Could you check a few things on this model? Use its own coordinates, in mm. A direction names the side the tool comes from. Give positions to 0.01 mm unless a question says otherwise; leave off trailing zeros. Loops run counter-clockwise (first coordinate to the right, second up) from the corner with the lowest first, then second, coordinate; pieces in that order, holes last. Notation, with made-up numbers: M 39,85 L 50,85 A11 cw 50,90 Z; hole C 10.5,6.25 d2. An arc over 180 degrees is marked long. Use CSV: the item, a comma, the result in double quotes.
Autodesk Inventor part; units mm, degrees
ref_plane "Work Plane1" through (0, -7, 0) normal (0, -1, 0) x (1, 0, 0)
ref_plane "YZ Plane" through (0, 0, 0) normal (1, 0, 0) x (0, 1, 0)
ref_plane "XZ Plane" through (0, 0, 0) normal (0, 1, 0) x (-1, 0, 0)
sketch "Sketch1" plane through (0, 0, 0) normal (0, 1, 0) x (-1, 0, 0)
  line L0 (0, 0) -> (3, 0)
  line L1 (3, 0) -> (3, -3)
  line L2 (0, 0) -> (-48.04, 0)
  line L3 (-48.04, 0) -> (-54, 0)
  line L4 (3, -3) -> (-54, -3)
  line L5 (-54, -3) -> (-54, 45)
  line L6 (-54, 45) -> (3, 45)
  line L7 (3, 45) -> (3, -3)
  line L8 (3, 21) -> (6.1215, 21)
  circle A0 centre (0, 0) radius 1.65
  circle A1 centre (-48.04, 0) radius 1.65
  line L9 (0, 42) -> (-48.04, 42)
  circle A2 centre (0, 42) radius 1.65
  circle A3 centre (-48.04, 42) radius 1.65
  line L10 (-54, -3) -> (-54, 8.785)
  line L11 (-54, 8.785) -> (-9.9, 8.785)
  line L12 (-9.9, 8.785) -> (-9.9, 23.785)
  line L13 (-9.9, 23.785) -> (-54, 23.785)
  dimension "d0" = 3
  dimension "d1" = 3
  dimension "d2" = 48.04
  dimension "d3" = 5.96
  dimension "d4" = 48
  dimension "d5" = 3.3
  dimension "d6" = 3.3
  dimension "d7" = 11.785
  dimension "d8" = 44.1
  dimension "d9" = 15
extrude "Extrusion1" add sketch "Sketch1" along normal blind 2 contours A0 L2 A1 L3 L5 L11 L12 L13 L6 L7 L0 | L0 L1 L4 L5 L3 A1 L2 A0
sketch "Sketch2" plane through (0, 0, 0) normal (0, -1, 0) x (1, 0, 0)
  line L0 (-3, -3) -> (-3, 45)
  line L1 (-3, -3) -> (-3, 5)
  line L2 (54, 8.785) -> (54, -3)
  line L3 (9.9, 8.785) -> (54, 8.785)
  line L4 (54, 8.785) -> (54, 4.785)
  line L5 (54, 8.785) -> (54, -3)
  line L6 (54, 23.785) -> (54, 27.785)
  line L7 (54, 45) -> (54, 23.785)
  line L8 (54, 27.785) -> (-3, 27.785)
  line L9 (-3, 5) -> (-3, 27.785)
  line L10 (9.9, 8.785) -> (54, 8.785)
  line L11 (54, 8.785) -> (9.9, 8.785)
  line L12 (9.9, 23.785) -> (9.9, 8.785)
  line L13 (9.9, 8.785) -> (9.9, 23.785)
  line L14 (9.9, 23.785) -> (54, 23.785)
  line L15 (-3, 5) -> (-3, 27.785)
  line L16 (-3, 27.785) -> (54, 27.785)
  line L17 (54, 27.785) -> (54, 4.785)
  line L18 (54, 4.785) -> (-3, 4.785)
  line L19 (-3, 4.785) -> (-3, 27.785)
  point P0 (0, 0)
  point P1 (-3, 4.785)
  dimension "d12" = 8
  dimension "d13" = 4
  dimension "d14" = 4
ref_plane "Work Plane1" through (0, -7, 0) normal (0, -1, 0) x (1, 0, 0)
sketch "Sketch4" plane through (54, 0, -3) normal (1, 0, 0) x (0, 0, -1)
  line L0 (-7.785, 0) -> (-7.785, -7)
  line L1 (-7.785, 0) -> (-7.785, 2)
  line L2 (0, 2) -> (-48, 2)
  line L3 (-7.785, 2) -> (-7.785, 15)
  line L4 (-30.785, 0) -> (-30.785, -7)
  line L5 (-30.785, 0) -> (-30.785, 15)
  line L6 (-7.785, 15) -> (-30.785, 15)
  line L7 (-26.785, -5) -> (-11.785, -5)
  line L8 (-11.785, 0) -> (-11.785, 2)
  line L9 (-11.785, -5) -> (-11.785, 2)
  line L10 (-11.785, 2) -> (-11.785, 13)
  line L11 (-26.785, 0) -> (-26.785, 2)
  line L12 (-26.785, 2) -> (-26.785, 13)
  line L13 (-26.785, 13) -> (-11.785, 13)
  point P0 (-3, 0)
  point P1 (-30.785, 2)
  dimension "d19" = 13
  dimension "d20" = 15
  dimension "d21" = 11
  dimension "d22" = 11
extrude "Extrusion5" add sketch "Sketch2" along normal blind 7 contours L0 L8 L6 L14 L12 L3 L2 L18
sketch "Sketch5" plane through (0, -7, 0) normal (0, -1, 0) x (1, 0, 0)
  line L0 (9.9, 23.785) -> (54, 23.785)
  line L1 (54, 23.785) -> (9.9, 23.785)
  line L2 (9.9, 23.785) -> (9.9, 8.785)
  line L3 (9.9, 8.785) -> (54, 8.785)
  line L4 (54, 8.785) -> (54, 23.785)
  point P0 (0, 0)
extrude "Extrusion6" add sketch "Sketch5" against normal blind 2
extrude "Extrusion7" add sketch "Sketch4" against normal blind 44.1 contours L2 L10 L13 L12 L5 L6 L3
sketch "Sketch6" plane through (9.9, 0, -3) normal (-1, 0, 0) x (0, 0, 1)
  line L0 (7.785, 15) -> (7.785, 2)
  line L1 (48, 2) -> (30.785, 2)
  line L2 (7.785, 15) -> (30.785, 15)
  line L3 (30.785, 15) -> (30.785, 2)
  line L4 (30.785, 2) -> (7.785, 2)
  line L5 (7.785, 2) -> (7.785, 15)
  point P0 (3, 0)
extrude "Extrusion8" add sketch "Sketch6" along normal blind 12.9
sketch "Sketch8" plane through (9.9, -5, 8.785) normal (0, 0, 1) x (1, 0, 0)
  line L0 (44.1, 0) -> (44.1, 18)
  line L1 (44.1, 0) -> (18.5, 0)
  line L2 (0, 0) -> (44.1, 0)
  line L3 (18.5, 0) -> (5.5, 0)
  line L4 (5.5, 0) -> (5.5, 1)
  line L5 (-12.9, 5) -> (44.1, 5)
  line L6 (5.5, 1) -> (14.6, 1)
  line L7 (44.1, -2) -> (-12.9, -2)
  line L8 (44.1, 18) -> (0, 18)
  line L9 (14.6, -2) -> (36.6, -2) construction
  line L10 (5.5, 1) -> (5.5, 18)
  line L11 (5.5, 18) -> (14.6, 18)
  line L12 (44.1, 18) -> (0, 18)
  line L13 (5.5, 1) -> (5.5, 17)
  line L14 (5.5, 17) -> (14.6, 17)
  line L15 (5.5, 17) -> (18.5, 17)
  line L16 (18.5, 17) -> (18.5, 1)
  line L17 (18.5, 1) -> (5.5, 1)
  point P0 (-9.9, 5)
  point P1 (5.5, 5)
  point P2 (14.6, 1)
  dimension "d33" = 25.6
  dimension "d34" = 13
  dimension "d35" = 1
  dimension "d39" = 16
  dimension "d42" = 13
extrude "Extrusion10" cut sketch "Sketch8" against normal blind 12.9 contours L16 L17 L6 L10 L5 | L5 L10 L14 L15 L16
sketch "Sketch11" plane through (0, 2, 0) normal (0, 1, 0) x (1, 0, 0)
  circle A0 centre (48.04, 0) radius 1.65
  circle A1 centre (0, 0) radius 1.65
  line L0 (48.04, 0) -> (0, 0)
  line L1 (24.02, 0) -> (24.02, 5.2317)
  line L2 (24.02, 0) -> (10.02, 0)
  line L3 (10.02, 0) -> (38.02, 0)
  line L4 (38.02, 0) -> (38.02, 7.5339)
  line L5 (54, -4.785) -> (-3, -4.785)
  line L6 (38.02, 7.5339) -> (10.02, 7.5339)
  line L7 (10.02, 7.5339) -> (10.02, -4.785)
  line L8 (10.02, -4.785) -> (38.02, -4.785)
  line L9 (38.02, -4.785) -> (38.02, 7.5339)
  dimension "d74" = 14
  dimension "d75" = 28
extrude "Extrusion12" cut sketch "Sketch11" against normal blind 10 contours L9 L5 L7 L0 | L0 L7 L6 L4
chamfer "Chamfer9" distance 7.785 angle 45 2 edges at (38.02, 1, -3) (10.02, 1, -3)
sketch "Sketch12" plane through (54, 13, 8.785) normal (0, -1, 0) x (1, 0, 0)
  line L0 (0, 0) -> (-44.1, 0)
  line L1 (-44.1, 0) -> (-44.1, 15)
  line L2 (0, 0) -> (-44.1, 0)
  line L3 (-44.1, 0) -> (-44.1, 15)
  line L4 (-44.1, 15) -> (0, 15)
  line L5 (0, 15) -> (0, 0)
  point P0 (-54, -8.785)
extrude "Extrusion13" cut sketch "Sketch12" against normal blind 0.125
sketch "Sketch13" plane through (0, -5, 0) normal (0, 1, 0) x (1, 0, 0)
  line L0 (54, -23.785) -> (9.9, -23.785)
  line L1 (9.9, -8.785) -> (54, -8.785)
  line L2 (54, -8.785) -> (54, -23.785)
  line L3 (54, -23.785) -> (9.9, -23.785)
  line L4 (9.9, -23.785) -> (9.9, -8.785)
  point P0 (0, 0)
extrude "Extrusion14" cut sketch "Sketch13" against normal blind 0.125
sketch "Sketch14" plane through (54, 13.125, 23.785) normal (0, 0, -1) x (-1, 0, 0)
  line L0 (44.1, -18.25) -> (44.1, 0)
  line L1 (0, -18.25) -> (44.1, -18.25)
  line L2 (44.1, 0) -> (0, 0)
  line L3 (0, 0) -> (0, -18.25)
  line L4 (0, -18.25) -> (44.1, -18.25)
  line L5 (44.1, -18.25) -> (44.1, 0)
  point P0 (54, -13.125)
extrude "Extrusion15" cut sketch "Sketch14" against normal blind 0.05
sketch "Sketch15" plane through (9.9, 13.125, 8.785) normal (0, 0, 1) x (1, 0, 0)
  line L0 (44.1, 0) -> (0, 0)
  line L1 (44.1, 0) -> (44.1, -18.25)
  line L2 (0, 0) -> (44.1, 0)
  line L3 (44.1, 0) -> (44.1, -18.25)
  line L4 (44.1, -18.25) -> (0, -18.25)
  line L5 (0, -18.25) -> (0, 0)
  point P0 (-9.9, -13.125)
extrude "Extrusion16" cut sketch "Sketch15" against normal blind 0.05
chamfer "Chamfer12" distance 9 angle 30 1 edges at (25.5, 2, 27.785) measured on face at (32.6017, 2, 32.1586)
chamfer "Chamfer13" distance 9 angle 30 1 edges at (25.5, 0, 27.785) measured on face at (32.6017, 0, 32.1586)
properties part number "U2D2 Plate"
1. Please list where these lines run through material, in increasing order: line 1 (Z direction, x = 0, y = 0.75); line 2 (Y direction, x = 30, z = 20) (3 decimals); line 3 (Z direction, x = 48.04, y = 1.45) (3 decimals).
Outcome:
line 1,"-3 to -1.65, 1.65 to 40.35, 43.65 to 45"
line 2,"-7 to -5.125, 13.125 to 15"
line 3,"-3 to -1.65, 1.65 to 8.735, 23.835 to 40.35, 43.65 to 45"
2. I want a section at A-A, the plane x = 12.5. List the corners of the cut face in (y, z) for me (3 decimals), then the cut area to 3 significant figures.
Outcome:
outline,"M -7,4.785 L 15,4.785 L 15,27.785 L 7.196,27.785 L 2,36.785 L 2,45 L 0,45 L 0,36.785 L -5.196,27.785 L -7,27.785 Z; hole M -5.125,8.735 L 13.125,8.735 L 13.125,23.835 L -5.125,23.835 Z"
area,"312 mm2"
3. Which directions (+Z, -Z, +X, -X, +Y, -Y) give clear straight access to the entire face, cutting with the end or side of a thin tool? Please do faces 1 (the face through (2, 0, 2)), 2 (the face through (32, -5.125, 16)), 3 (the face through (26, -6, 27.785)).
Outcome:
face 1,"-Z, +X, -X, -Y"
face 2,"+X"
face 3,"+Z, +X, -X, -Y"
4. If we mould it in two halves opening along Y, with no side actions, what happens to faces 4 (the face through (26, 1, 45)), 5 (the face through (25, -7, 16)), 6 (the face through (37, 4, 8.735))? For each: +Y half, -Y half, draft (parallel to the pull), parting line (faces both ways), or undercut.
Outcome:
face 4,"draft"
face 5,"-Y half"
face 6,"undercut"
5. I'm going to push flat-ended pins straight in: pin 1 Ø2 at (x, z) = (3, 2.5) entering from -Y; pin 2 Ø4 at (x, z) = (44.5, 1) entering from +Y; pin 3 Ø1.5 at (x, y) = (28.5, 6.5) entering from +Z; pin 4 Ø3 at (x, z) = (48.04, 42) entering from +Y. Where does each tip first touch, or does it pass through?
Outcome:
pin 1,"y = 0"
pin 2,"y = 2"
pin 3,"z = 30.29"
pin 4,"through"
6. I want a section at D-D, the plane y = 4. List the corners of the cut face in (x, z) for me (3 decimals), then the cut area to 3 significant figures.
Outcome:
outline,"M -3,4.785 L 15.4,4.785 L 15.4,8.735 L 9.9,8.735 L 9.9,23.835 L 54,23.835 L 54,33.321 L -3,33.321 Z; M 28.4,4.785 L 54,4.785 L 54,8.735 L 28.4,8.735 Z"
area,"909 mm2"
7. I want a section at B-B, the plane z = 42. List the corners of the cut face in (x, y) for me.
Outcome:
outline,"M -3,0 L -1.65,0 L -1.65,2 L -3,2 Z; M 1.65,0 L 46.39,0 L 46.39,2 L 1.65,2 Z; M 49.69,0 L 54,0 L 54,2 L 49.69,2 Z"
8. I want a section at C-C, the plane x = 48.04. List the corners of the cut face in (y, z) for me (3 decimals), then the cut area to 3 significant figures.
Outcome:
outline,"M -7,4.785 L 0,4.785 L 0,1.65 L 2,1.65 L 2,4.785 L 15,4.785 L 15,27.785 L 7.196,27.785 L 2,36.785 L 2,40.35 L 0,40.35 L 0,36.785 L -5.196,27.785 L -7,27.785 Z; M 0,-3 L 2,-3 L 2,-1.65 L 0,-1.65 Z; M 0,43.65 L 2,43.65 L 2,45 L 0,45 Z; hole M -5.125,8.735 L 13.125,8.735 L 13.125,23.835 L -5.125,23.835 Z"
area,"314 mm2"
